Could you check a few things on this model? Use its own coordinates, in mm. Face numbers are marked on the shaded views. A direction names the side the tool comes from. Coordinates: 2 decimals unless noted, no trailing zeros. Loops run counter-clockwise (first coordinate to the right, second up) from the corner with the lowest first, then second, coordinate; pieces in that order, holes last.
1) If I drill on line 1 along X through (y, z) = (3.25, 54.5); line 2 along Z through (x, y) = (-3.5, 6); line 3 along Y through (x, z) = (-5.5, 25) (3 decimals), over which ranges is the centre line in solid material (lowest first)?
2) For the marked faces 1 and 2, which set-ups out of +Z, -Z, +X, -X, +Y, -Y let a thin tool reach every point of the face, with its end or its side?
3) Thinking about a two-plate mould opening in X: for the marked faces 3, 4 and 5, which applies, released by +X, released by -X, zero draft, split by the parting line, or undercut?
4) Will these pins go through, and if not, where does the flat tip stop? P1, Ø2.5, axis at x = -4, z = 6, coming from the +Y side (3 decimals); P2, Ø0.8, axis at x = -37.5, z = 19, coming from the +Y side; P3, Ø0.8, axis at x = -37, z = 9, coming from the +Y side.
5) Imagine slicing it at A-A on x = -32.5. Please give me the cut outline in (y, z) (1 decimal).
6) Imagine slicing it at C-C on y = 12. Give the number of separate pieces and of enclosed holes in the cut face, plus the area to 3 significant figures.
7) Imagine slicing it at D-D on x = -19.5. Please give me the cut outline in (y, z) (1 decimal).
8) Imagine slicing it at B-B on z = 49.5. Please give me the cut outline in (x, y) (1 decimal).
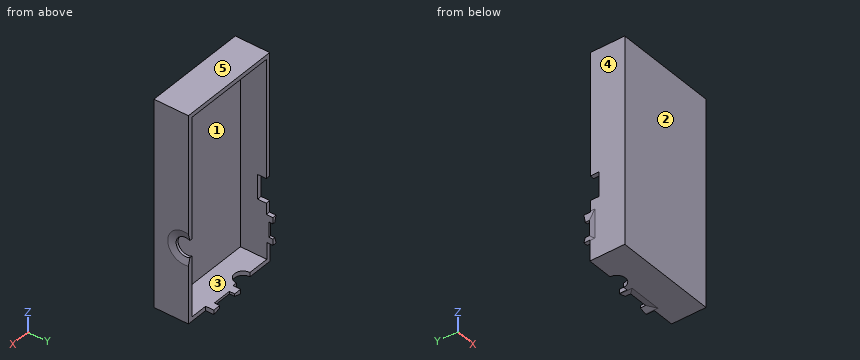
```python
from build123d import *

# Parameters (mm, degrees)
SKETCH1_W           = 38.1
SKETCH1_H           = 76.2
BOSS_EXTRUDE1_DEPTH = 15.875
SKETCH4_W           = 34.925
SKETCH4_H           = 73.025
CUT_EXTRUDE2_DEPTH  = 12.7
CUT_EXTRUDE3_DEPTH  = 1.5875
CHAMFER1_SIZE       = 2.54
CHAMFER1_SIZE2      = 0.680590949
CUT_EXTRUDE4_DEPTH  = 1.5875
CHAMFER2_SIZE       = 2.54
CHAMFER2_SIZE2      = 0.680590949
SKETCH7_W           = 34.925
SKETCH7_H           = 3.175
CUT_EXTRUDE5_DEPTH  = 1.5875
CUT_EXTRUDE6_DEPTH  = 1.5875


with BuildPart() as part:
    # Sketch1 → Boss-Extrude1 (new body)
    with BuildSketch(Plane(origin=(0, 0, 0), x_dir=(1, 0, 0), z_dir=(0, 1, 0))):
        with Locations((-19.05, -38.1)):
            Rectangle(SKETCH1_W, SKETCH1_H)
    extrude(amount=BOSS_EXTRUDE1_DEPTH)

    # Sketch4 → Cut-Extrude2 (cut)
    with BuildSketch(Plane(origin=(0, 15.875, 0), x_dir=(1, 0, 0), z_dir=(0, 1, 0))):
        with Locations((-19.05, -38.1)):
            Rectangle(SKETCH4_W, SKETCH4_H)
    extrude(amount=-CUT_EXTRUDE2_DEPTH, mode=Mode.SUBTRACT)

    # Sketch5 → Cut-Extrude3 (cut)
    with BuildSketch(Plane(origin=(0, 0, 0), x_dir=(0, 0, -1), z_dir=(1, 0, 0))):
        with BuildLine():
            Line((0, 12.7), (-23.851432546, 12.7))
            ThreePointArc((-23.851432546, 12.7), (-26.9833, 7.6375), (-30.115167454, 12.7))
            Line((-30.115167454, 12.7), (-76.2, 12.7))
            Line((-76.2, 12.7), (-76.2, 15.875))
            Line((-76.2, 15.875), (0, 15.875))
            Line((0, 15.875), (0, 12.7))
        make_face()
    extrude(amount=-CUT_EXTRUDE3_DEPTH, mode=Mode.SUBTRACT)

    # Chamfer1
    chamfer1_edges = [part.edges().sort_by_distance(p)[0] for p in [
        (0, 7.6375, 26.9833),
    ]]
    chamfer1_side = [part.faces().sort_by_distance(p)[0] for p in [
        (0, 6.21970244, 38.453254935),
    ]]
    chamfer(chamfer1_edges, length=CHAMFER1_SIZE, length2=CHAMFER1_SIZE2, reference=chamfer1_side[0])

    # Sketch6 → Cut-Extrude4 (cut)
    with BuildSketch(Plane(origin=(0, 0, 0), x_dir=(-1, 0, 0), z_dir=(0, 0, -1))):
        with BuildLine():
            Line((1.5875, 12.7), (8.0883, 12.7))
            Line((8.0883, 12.7), (8.0883, 15.6875))
            Line((8.0883, 15.6875), (10.8883, 15.6875))
            Line((10.8883, 15.6875), (10.8883, 13.7375))
            Line((10.8883, 13.7375), (17.8883, 13.7375))
            Line((17.8883, 13.7375), (17.8883, 15.6875))
            Line((17.8883, 15.6875), (20.6883, 15.6875))
            Line((20.6883, 15.6875), (20.6883, 12.8725))
            Line((20.6883, 12.8725), (22.2783, 12.8725))
            ThreePointArc((22.2783, 12.8725), (25.4533, 9.6975), (28.6283, 12.8725))
            Line((28.6283, 12.8725), (38.1, 12.8725))
            Line((38.1, 12.8725), (38.1, 15.875))
            Line((38.1, 15.875), (1.5875, 15.875))
            Line((1.5875, 15.875), (1.5875, 12.7))
        make_face()
    extrude(amount=-CUT_EXTRUDE4_DEPTH, mode=Mode.SUBTRACT)

    # Chamfer2
    chamfer2_edges = [part.edges().sort_by_distance(p)[0] for p in [
        (-10.8883, 14.7125, 0),
        (-14.3883, 13.7375, 0),
        (-17.8883, 14.7125, 0),
    ]]
    chamfer2_side = [part.faces().sort_by_distance(p)[0] for p in [
        (-18.682001646, 6.589374137, 0),
    ]]
    chamfer(chamfer2_edges, length=CHAMFER2_SIZE, length2=CHAMFER2_SIZE2, reference=chamfer2_side[0])

    # Sketch7 → Cut-Extrude5 (cut)
    with BuildSketch(Plane.XY.offset(76.2)):
        with Locations((-19.05, 14.2875)):
            Rectangle(SKETCH7_W, SKETCH7_H)
    extrude(amount=-CUT_EXTRUDE5_DEPTH, mode=Mode.SUBTRACT)

    # Sketch8 → Cut-Extrude6 (cut)
    with BuildSketch(Plane.ZY.offset(38.1)):
        Polygon((76.2, 12.7), (31.0375, 12.7), (31.0375, 9.525), (22.0375, 9.525), (22.0375, 12.7), (17.913122854, 12.7), (17.913122854, 15.0975), (15.633122854, 15.0975), (15.633122854, 13.5975), (10.038122854, 13.5975), (10.033122854, 15.0975), (7.753122854, 15.0975), (7.753122854, 12.8725), (1.5875, 12.8725), (1.5875, 15.875), (76.2, 15.875), align=None)
    extrude(amount=-CUT_EXTRUDE6_DEPTH, mode=Mode.SUBTRACT)

    # Chamfer3
    # the kernel refuses this chamfer: 2.54, 0.680590949 mm, written as the material it takes off along each edge
    with BuildSketch(Plane(origin=(-38.1, 7.001863854, 10.060108308), x_dir=(-0.009967146577155543, -0.003333149238426835, -0.9999447715275398), z_dir=(0, 0.9999944444907404, -0.003333314814970836))) as chamfer3_piece_1_section:
        with BuildLine():
            Line((2.638269115, 0), (-0.105178835, -0.705873694))
            Line((-0.105178835, -0.705873694), (-0.155976312, -0.705367363))
            ThreePointArc((-0.155976312, -0.705367363), (-0.0543203, -0.352919594), (-0.050797477, 0.000506331))
            Line((-0.050797477, 0.000506331), (0.000506331, 0.050797477))
            ThreePointArc((0.000506331, 0.050797477), (1.319509841, 0.037650122), (2.638775446, 0.050797477))
            Line((2.638775446, 0.050797477), (2.638269115, 0))
        make_face()
    chamfer3_piece_1 = extrude(amount=14.69135391, mode=Mode.PRIVATE)
    chamfer3_piece_1 = split(chamfer3_piece_1, bisect_by=Plane(origin=(-37.899401738, 15.0975, 9.151337031), z_dir=(0, -1, 0)), keep=Keep.TOP, mode=Mode.PRIVATE)
    chamfer3_piece_1 = split(chamfer3_piece_1, bisect_by=Plane(origin=(-37.899401738, 13.5975, 9.151337031), z_dir=(0, 1, 0)), keep=Keep.TOP, mode=Mode.PRIVATE)
    add(chamfer3_piece_1, mode=Mode.SUBTRACT)
    with BuildSketch(Plane(origin=(-38.1, 13.5975, 15.633122854), x_dir=(-0.009967146577155547, -0.9999503267608394, 0), z_dir=(0, 0, -1))) as chamfer3_piece_2_section:
        with BuildLine():
            Line((2.638269115, 0), (-0.105178835, -0.705873694))
            Line((-0.105178835, -0.705873694), (-0.155976312, -0.705367363))
            ThreePointArc((-0.155976312, -0.705367363), (-0.0543203, -0.352919594), (-0.050797477, 0.000506331))
            Line((-0.050797477, 0.000506331), (0.000506331, 0.050797477))
            ThreePointArc((0.000506331, 0.050797477), (1.319509841, 0.037650122), (2.638775446, 0.050797477))
            Line((2.638775446, 0.050797477), (2.638269115, 0))
        make_face()
    chamfer3_piece_2 = extrude(amount=12.190672788, mode=Mode.PRIVATE)
    chamfer3_piece_2 = split(chamfer3_piece_2, bisect_by=Plane(origin=(-37.899362184, 12.704169113, 10.041100623), z_dir=(0, 0.003333314814970836, 0.9999944444907404)), keep=Keep.TOP, mode=Mode.PRIVATE)
    add(chamfer3_piece_2, mode=Mode.SUBTRACT)
    with BuildSketch(Plane(origin=(-38.1, 15.0975, 15.633122854), x_dir=(-0.009967146577155547, -2.3683581360028347e-15, 0.9999503267608394), z_dir=(0, -1, 0))) as chamfer3_piece_3:
        with BuildLine():
            Line((2.638269115, 0), (-0.105178835, -0.705873694))
            Line((-0.105178835, -0.705873694), (-0.155976312, -0.705367363))
            ThreePointArc((-0.155976312, -0.705367363), (-0.0543203, -0.352919594), (-0.050797477, 0.000506331))
            Line((-0.050797477, 0.000506331), (0.000506331, 0.050797477))
            ThreePointArc((0.000506331, 0.050797477), (1.319509841, 0.037650122), (2.638775446, 0.050797477))
            Line((2.638775446, 0.050797477), (2.638269115, 0))
        make_face()
    extrude(amount=1.5, mode=Mode.SUBTRACT)
    with BuildSketch(Plane(origin=(-38.1, 7.001863854, 10.060108308), x_dir=(-0.009967146577155543, -0.003333149238426835, -0.9999447715275398), z_dir=(0, 0.9999944444907404, -0.003333314814970836))) as chamfer3_piece_4a_section:
        with BuildLine():
            Line((2.638269115, 0), (-0.105178835, -0.705873694))
            Line((-0.105178835, -0.705873694), (-0.155976312, -0.705367363))
            ThreePointArc((-0.155976312, -0.705367363), (-0.0543203, -0.352919594), (-0.050797477, 0.000506331))
            Line((-0.050797477, 0.000506331), (0.000506331, 0.050797477))
            ThreePointArc((0.000506331, 0.050797477), (1.319509841, 0.037650122), (2.638775446, 0.050797477))
            Line((2.638775446, 0.050797477), (2.638269115, 0))
        make_face()
    chamfer3_piece_4a = extrude(amount=14.69135391, mode=Mode.PRIVATE)
    chamfer3_piece_4a = split(chamfer3_piece_4a, bisect_by=Plane(origin=(-37.899435258, 13.5975, 9.16460585), z_dir=(0, -1, 0)), keep=Keep.TOP, mode=Mode.PRIVATE)
    with BuildSketch(Plane(origin=(-38.1, 13.5975, 15.633122854), x_dir=(-0.009967146577155547, -0.9999503267608394, 0), z_dir=(0, 0, -1))) as chamfer3_piece_4b_section:
        with BuildLine():
            Line((2.638269115, 0), (-0.105178835, -0.705873694))
            Line((-0.105178835, -0.705873694), (-0.155976312, -0.705367363))
            ThreePointArc((-0.155976312, -0.705367363), (-0.0543203, -0.352919594), (-0.050797477, 0.000506331))
            Line((-0.050797477, 0.000506331), (0.000506331, 0.050797477))
            ThreePointArc((0.000506331, 0.050797477), (1.319509841, 0.037650122), (2.638775446, 0.050797477))
            Line((2.638775446, 0.050797477), (2.638269115, 0))
        make_face()
    chamfer3_piece_4b = extrude(amount=12.190672788, mode=Mode.PRIVATE)
    chamfer3_piece_4b = split(chamfer3_piece_4b, bisect_by=Plane(origin=(-37.899435258, 12.723987849, 10.041034561), z_dir=(0, -0.003333314814970836, -0.9999944444907404)), keep=Keep.TOP, mode=Mode.PRIVATE)
    chamfer3_piece_4 = chamfer3_piece_4a & chamfer3_piece_4b
    add(chamfer3_piece_4, mode=Mode.SUBTRACT)
    with BuildSketch(Plane(origin=(-38.1, 13.5975, 22.228795642), x_dir=(-0.00996714657715554, -0.9999503267608394, 0), z_dir=(0, 0, -1))) as chamfer3_piece_5a_section:
        with BuildLine():
            Line((2.638269115, 0), (-0.105178835, -0.705873694))
            Line((-0.105178835, -0.705873694), (-0.155976312, -0.705367363))
            ThreePointArc((-0.155976312, -0.705367363), (-0.0543203, -0.352919594), (-0.050797477, 0.000506331))
            Line((-0.050797477, 0.000506331), (0.000506331, 0.050797477))
            ThreePointArc((0.000506331, 0.050797477), (1.319509841, 0.037650122), (2.638775446, 0.050797477))
            Line((2.638775446, 0.050797477), (2.638269115, 0))
        make_face()
    chamfer3_piece_5a = extrude(amount=18.786345577, mode=Mode.PRIVATE)
    chamfer3_piece_5a = split(chamfer3_piece_5a, bisect_by=Plane(origin=(-37.899401738, 12.71321909, 15.633122854), z_dir=(0, 0, 1)), keep=Keep.TOP, mode=Mode.PRIVATE)
    with BuildSketch(Plane(origin=(-38.1, 15.0975, 15.633122854), x_dir=(-0.009967146577155547, -2.3683581360028347e-15, 0.9999503267608394), z_dir=(0, -1, 0))) as chamfer3_piece_5b_section:
        with BuildLine():
            Line((2.638269115, 0), (-0.105178835, -0.705873694))
            Line((-0.105178835, -0.705873694), (-0.155976312, -0.705367363))
            ThreePointArc((-0.155976312, -0.705367363), (-0.0543203, -0.352919594), (-0.050797477, 0.000506331))
            Line((-0.050797477, 0.000506331), (0.000506331, 0.050797477))
            ThreePointArc((0.000506331, 0.050797477), (1.319509841, 0.037650122), (2.638775446, 0.050797477))
            Line((2.638775446, 0.050797477), (2.638269115, 0))
        make_face()
    chamfer3_piece_5b = extrude(amount=8.095672788, mode=Mode.PRIVATE)
    chamfer3_piece_5b = split(chamfer3_piece_5b, bisect_by=Plane(origin=(-37.899401738, 13.5975, 16.517403764), z_dir=(0, -1, 0)), keep=Keep.TOP, mode=Mode.PRIVATE)
    chamfer3_piece_5 = chamfer3_piece_5a & chamfer3_piece_5b
    add(chamfer3_piece_5, mode=Mode.SUBTRACT)


solid = part.part
```
Filled in:
1. line 1: x = -38.1 to -36.51, -1.59 to 0
1. line 2: z = 0 to 1.59, 74.61 to 76.2
1. line 3: y = 0 to 3.175
2. face 1: +Y
2. face 2: +Z, -Z, +X, -X, -Y
3. face 3: undercut
3. face 4: released by -X
3. face 5: zero draft
4. P1: stops at y = 3.175
4. P2: stops at y = 12.7
4. P3: stops at y = 15.1
5. outline: (0, 0) - (12.9, 0) - (12.9, 1.6) - (3.2, 1.6) - (3.2, 74.6) - (12.7, 74.6) - (12.7, 76.2) - (0, 76.2) - close
6. separate pieces: 3
6. enclosed holes: 0
6. area: 311 mm2
7. outline: (0, 0) - (11.2, 0) - (12.1, 0.2) - (15.7, 0.2) - (15.7, 1.6) - (3.2, 1.6) - (3.2, 74.6) - (12.7, 74.6) - (12.7, 76.2) - (0, 76.2) - close
8. outline: (-38.1, 0) - (0, 0) - (0, 12.7) - (-1.6, 12.7) - (-1.6, 3.2) - (-36.5, 3.2) - (-36.5, 12.7) - (-38.1, 12.7) - close
